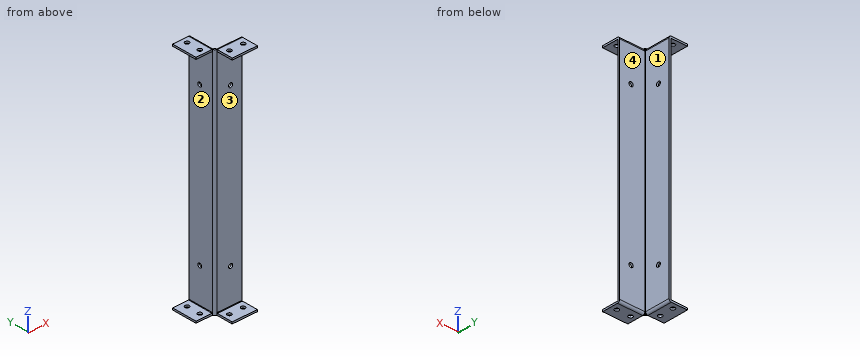
```python
from build123d import *

# Parameters (mm, degrees)
SKETCH1_W                      = 60
SKETCH1_H                      = 500.5
BASE_FLANGE1_DEPTH             = 4
EDGE_FLANGE1_STRIP_W           = 18
EDGE_FLANGE1_STRIP_H           = 4
EDGE_FLANGE1_STRIP_CUT_DEPTH   = 500.5
EDGE_FLANGE1_DEPTH             = 500.5
EDGE_FLANGE2_STRIP_W           = 18
EDGE_FLANGE2_STRIP_H           = 4
EDGE_FLANGE2_STRIP_CUT_DEPTH   = 55
EDGE_FLANGE2_STRIP_2_W         = 18
EDGE_FLANGE2_STRIP_2_H         = 4
EDGE_FLANGE2_STRIP_CUT_2_DEPTH = 55
EDGE_FLANGE2_STRIP_3_W         = 18
EDGE_FLANGE2_STRIP_3_H         = 4
EDGE_FLANGE2_STRIP_CUT_3_DEPTH = 55
EDGE_FLANGE2_STRIP_4_W         = 18
EDGE_FLANGE2_STRIP_4_H         = 4
EDGE_FLANGE2_STRIP_CUT_4_DEPTH = 55
EDGE_FLANGE2_DEPTH             = 55
EDGE_FLANGE2_BEND_DEPTH        = 55
EDGE_FLANGE2_BEND_2_DEPTH      = 55
EDGE_FLANGE2_BEND_3_DEPTH      = 55
SKETCH18_R                     = 4.6
EXTRUDE1_DEPTH                 = 509.385926241
SKETCH19_R                     = 4.6
EXTRUDE2_DEPTH                 = 4
SKETCH20_R                     = 4.6
EXTRUDE3_DEPTH                 = 4


# Sheet-metal steps are written as plain solids
with BuildPart() as part:
    # Sketch1 → Base-Flange1 (new body)
    with BuildSketch(Plane(origin=(0, 0, 0), x_dir=(1, 0, 0), z_dir=(0, 1, 0))):
        Rectangle(SKETCH1_W, SKETCH1_H)
    extrude(amount=BASE_FLANGE1_DEPTH)

    # Edge-Flange1 strip (across the edge) → Edge-Flange1 strip cut (cut)
    with BuildSketch(Plane(origin=(-30, 4, -250.25), x_dir=(1, 0, 0), z_dir=(0, 0, 1))):
        with Locations((-4, -2)):
            Rectangle(EDGE_FLANGE1_STRIP_W, EDGE_FLANGE1_STRIP_H)
    extrude(amount=EDGE_FLANGE1_STRIP_CUT_DEPTH, mode=Mode.SUBTRACT)

    # Edge-Flange1 section (across the edge) → Edge-Flange1 (add)
    with BuildSketch(Plane(origin=(-30, 4, -250.25), x_dir=(1, 0, 0), z_dir=(0, 0, 1))):
        with BuildLine():
            Line((0, 1), (0, 56))
            Line((0, 56), (4, 56))
            Line((4, 56), (4, 1))
            ThreePointArc((4, 1), (4.292893219, 0.292893219), (5, 0))
            Line((5, 0), (5, -4))
            ThreePointArc((5, -4), (1.464466094, -2.535533906), (0, 1))
        make_face()
    extrude(amount=EDGE_FLANGE1_DEPTH)

    # Edge-Flange2 strip (across the edge) → Edge-Flange2 strip cut (cut)
    with BuildSketch(Plane(origin=(-30, 5, 250.25), x_dir=(0, 0, -1), z_dir=(0, 1, 0))):
        with Locations((-4, -2)):
            Rectangle(EDGE_FLANGE2_STRIP_W, EDGE_FLANGE2_STRIP_H)
    extrude(amount=EDGE_FLANGE2_STRIP_CUT_DEPTH, mode=Mode.SUBTRACT)

    # Edge-Flange2 strip 2 (across the edge) → Edge-Flange2 strip cut 2 (cut)
    with BuildSketch(Plane(origin=(30, 0, 250.25), x_dir=(0, 0, -1), z_dir=(-1, 0, 0))):
        with Locations((-4, -2)):
            Rectangle(EDGE_FLANGE2_STRIP_2_W, EDGE_FLANGE2_STRIP_2_H)
    extrude(amount=EDGE_FLANGE2_STRIP_CUT_2_DEPTH, mode=Mode.SUBTRACT)

    # Edge-Flange2 strip 3 (across the edge) → Edge-Flange2 strip cut 3 (cut)
    with BuildSketch(Plane(origin=(-30, 60, -250.25), x_dir=(0, 0, 1), z_dir=(0, -1, 0))):
        with Locations((-4, -2)):
            Rectangle(EDGE_FLANGE2_STRIP_3_W, EDGE_FLANGE2_STRIP_3_H)
    extrude(amount=EDGE_FLANGE2_STRIP_CUT_3_DEPTH, mode=Mode.SUBTRACT)

    # Edge-Flange2 strip 4 (across the edge) → Edge-Flange2 strip cut 4 (cut)
    with BuildSketch(Plane(origin=(-25, 0, -250.25), x_dir=(0, 0, 1), z_dir=(1, 0, 0))):
        with Locations((-4, -2)):
            Rectangle(EDGE_FLANGE2_STRIP_4_W, EDGE_FLANGE2_STRIP_4_H)
    extrude(amount=EDGE_FLANGE2_STRIP_CUT_4_DEPTH, mode=Mode.SUBTRACT)

    # Edge-Flange2 section (across the edge) → Edge-Flange2 (add)
    with BuildSketch(Plane(origin=(-30, 5, 250.25), x_dir=(0, 0, -1), z_dir=(0, 1, 0))):
        with BuildLine():
            Line((0, 1), (0, 36))
            Line((0, 36), (4, 36))
            Line((4, 36), (4, 1))
            ThreePointArc((4, 1), (4.292893219, 0.292893219), (5, 0))
            Line((5, 0), (5, -4))
            ThreePointArc((5, -4), (1.464466094, -2.535533906), (0, 1))
        make_face()
    extrude(amount=EDGE_FLANGE2_DEPTH)

    # Edge-Flange2 section 2 (across the edge) → Edge-Flange2 bend (add)
    with BuildSketch(Plane(origin=(30, 0, 250.25), x_dir=(0, 0, -1), z_dir=(-1, 0, 0))):
        with BuildLine():
            Line((0, 1), (0, 36))
            Line((0, 36), (4, 36))
            Line((4, 36), (4, 1))
            ThreePointArc((4, 1), (4.292893219, 0.292893219), (5, 0))
            Line((5, 0), (5, -4))
            ThreePointArc((5, -4), (1.464466094, -2.535533906), (0, 1))
        make_face()
    extrude(amount=EDGE_FLANGE2_BEND_DEPTH)

    # Edge-Flange2 section 3 (across the edge) → Edge-Flange2 bend 2 (add)
    with BuildSketch(Plane(origin=(-30, 60, -250.25), x_dir=(0, 0, 1), z_dir=(0, -1, 0))):
        with BuildLine():
            Line((0, 1), (0, 36))
            Line((0, 36), (4, 36))
            Line((4, 36), (4, 1))
            ThreePointArc((4, 1), (4.292893219, 0.292893219), (5, 0))
            Line((5, 0), (5, -4))
            ThreePointArc((5, -4), (1.464466094, -2.535533906), (0, 1))
        make_face()
    extrude(amount=EDGE_FLANGE2_BEND_2_DEPTH)

    # Edge-Flange2 section 4 (across the edge) → Edge-Flange2 bend 3 (add)
    with BuildSketch(Plane(origin=(-25, 0, -250.25), x_dir=(0, 0, 1), z_dir=(1, 0, 0))):
        with BuildLine():
            Line((0, 1), (0, 36))
            Line((0, 36), (4, 36))
            Line((4, 36), (4, 1))
            ThreePointArc((4, 1), (4.292893219, 0.292893219), (5, 0))
            Line((5, 0), (5, -4))
            ThreePointArc((5, -4), (1.464466094, -2.535533906), (0, 1))
        make_face()
    extrude(amount=EDGE_FLANGE2_BEND_3_DEPTH)

    # Sketch18 → Extrude1 (cut, through all)
    with BuildSketch(Plane.XY.offset(250.25)):
        with Locations((-46, 47.5)):
            Circle(SKETCH18_R)
        with Locations((-46, 17.5)):
            Circle(SKETCH18_R)
        with Locations((-12.5, -16)):
            Circle(SKETCH18_R)
        with Locations((17.5, -16)):
            Circle(SKETCH18_R)
    extrude(amount=-EXTRUDE1_DEPTH, mode=Mode.SUBTRACT)

    # Sketch19 → Extrude2 (cut)
    with BuildSketch(Plane(origin=(-26, 0, 0), x_dir=(0, 0, -1), z_dir=(1, 0, 0))):
        with Locations(Location((-170.25, 35, 0), (0, 0, 90))):
            Circle(SKETCH19_R)
        with Locations(Location((170.25, 35, 0), (0, 0, 90))):
            Circle(SKETCH19_R)
    extrude(amount=-EXTRUDE2_DEPTH, mode=Mode.SUBTRACT)

    # Sketch20 → Extrude3 (cut)
    with BuildSketch(Plane(origin=(0, 4, 0), x_dir=(1, 0, 0), z_dir=(0, 1, 0))):
        with Locations(Location((5, 170.25, 0), (0, 0, 270))):
            Circle(SKETCH20_R)
        with Locations(Location((5, -170.25, 0), (0, 0, 270))):
            Circle(SKETCH20_R)
    extrude(amount=-EXTRUDE3_DEPTH, mode=Mode.SUBTRACT)


solid = part.part
```
Geometry check sheet. Reference: the model listing, model coordinates, mm. Face numbers are marked on the shaded views. A direction names the side the tool comes from. Give positions to 0.01 mm unless a question says otherwise; leave off trailing zeros. Order: outer loops, then holes, each group sorted by start corner. A loop starts at its lowest first (then second) coordinate and runs counter-clockwise, first axis right, second up.
1. Section check D-D, the plane x = -12.5. Enter the section's corners in (y, z).
2. Access from +Z, -Z, +X, -X, +Y, -Y to the whole of each face (thin tool, end or side, straight path). Record for the marked faces 1 and 2.
3. Section check C-C, the plane x = -46. Enter the section's corners in (y, z).
4. Gauge pin test, flat ends, axial feed: pin 1 Ø1 at (x, z) = (19.5, 14.5) entering from -Y; pin 2 Ø4 at (y, z) = (-25, -248.5) entering from -X; pin 3 Ø1 at (y, z) = (36.5, 130.5) entering from +X. Record the tip position at first contact, or that the pin passes through.
5. Section check B-B, the plane y = 17.5. Enter the section's corners in (x, z).
6. Thickness scan on L1, parallel to Y at x = -46, z = 247.15; L2, parallel to Z at x = 24.5, y = -21; L3, parallel to Z at x = -27.1, y = 35. Record the ranges inside material, lowest first.
7. Section check A-A, the plane z = 170.25. Enter the section's corners in (x, y), and give its area (3 significant figures).
8. Release check for a two-part mould opening along Z. For the marked faces 3 and 4 record: pulls with the +Z half, pulls with the -Z half, needs draft (parallel to the pull), parting line crosses it, or undercut.
Values follow:
1. outline: (-36, -250.25) - (-20.6, -250.25) - (-20.6, -246.25) - (-36, -246.25) - close; (-36, 246.25) - (-20.6, 246.25) - (-20.6, 250.25) - (-36, 250.25) - close; (-11.4, -250.25) - (-1, -250.25) arc R5 ccw to (4, -245.25) - (4, 245.25) arc R5 ccw to (-1, 250.25) - (-11.4, 250.25) - (-11.4, 246.25) - (-1, 246.25) arc R1 cw to (0, 245.25) - (0, -245.25) arc R1 cw to (-1, -246.25) - (-11.4, -246.25) - close
2. face 1: +Z, -Z, +X, +Y
2. face 2: -X, +Y, -Y
3. outline: (5, -250.25) - (12.9, -250.25) - (12.9, -246.25) - (5, -246.25) - close; (5, 246.25) - (12.9, 246.25) - (12.9, 250.25) - (5, 250.25) - close; (22.1, -250.25) - (42.9, -250.25) - (42.9, -246.25) - (22.1, -246.25) - close; (22.1, 246.25) - (42.9, 246.25) - (42.9, 250.25) - (22.1, 250.25) - close; (52.1, -250.25) - (60, -250.25) - (60, -246.25) - (52.1, -246.25) - close; (52.1, 246.25) - (60, 246.25) - (60, 250.25) - (52.1, 250.25) - close
4. pin 1: stops at y = 0
4. pin 2: stops at x = -25
4. pin 3: stops at x = -26
5. outline: (-66, -250.25) - (-50.6, -250.25) - (-50.6, -246.25) - (-66, -246.25) - close; (-66, 246.25) - (-50.6, 246.25) - (-50.6, 250.25) - (-66, 250.25) - close; (-41.4, -250.25) - (-31, -250.25) arc R5 ccw to (-26, -245.25) - (-26, 245.25) arc R5 ccw to (-31, 250.25) - (-41.4, 250.25) - (-41.4, 246.25) - (-31, 246.25) arc R1 cw to (-30, 245.25) - (-30, -245.25) arc R1 cw to (-31, -246.25) - (-41.4, -246.25) - close
6. L1: y = 5 to 12.9, 22.1 to 42.9, 52.1 to 60
6. L2: z = -250.25 to -246.25, 246.25 to 250.25
6. L3: z = -248.38 to -174.85, -165.65 to 165.65, 174.85 to 248.38
7. outline: (-30, 5) arc R5 ccw to (-25, 0) - (0.4, 0) - (0.4, 4) - (-25, 4) arc R1 cw to (-26, 5) - (-26, 30.4) - (-30, 30.4) - close; (-30, 39.6) - (-26, 39.6) - (-26, 60) - (-30, 60) - close; (9.6, 0) - (30, 0) - (30, 4) - (9.6, 4) - close
7. area: 385 mm2
8. face 3: undercut
8. face 4: needs draft
